The drawing under review shows one solid part. Ordinate dimensions are in mm from its lowest x, y, z. A direction names the side the tool comes from. Coordinates: 2 decimals unless noted, no trailing zeros. Order: outer loops, then holes, each group sorted by start corner. A loop starts at its lowest first (then second) coordinate and runs counter-clockwise, first axis right, second up. Notation, with made-up numbers: (-38, 25.25) -> (-15, 25.25) arc R27 ccw to (-15, 46.25) -> close; hole circle Ø1 at (-10.5, 40). An arc over 180 degrees is marked (long way). Use one line per item in the form item = value.
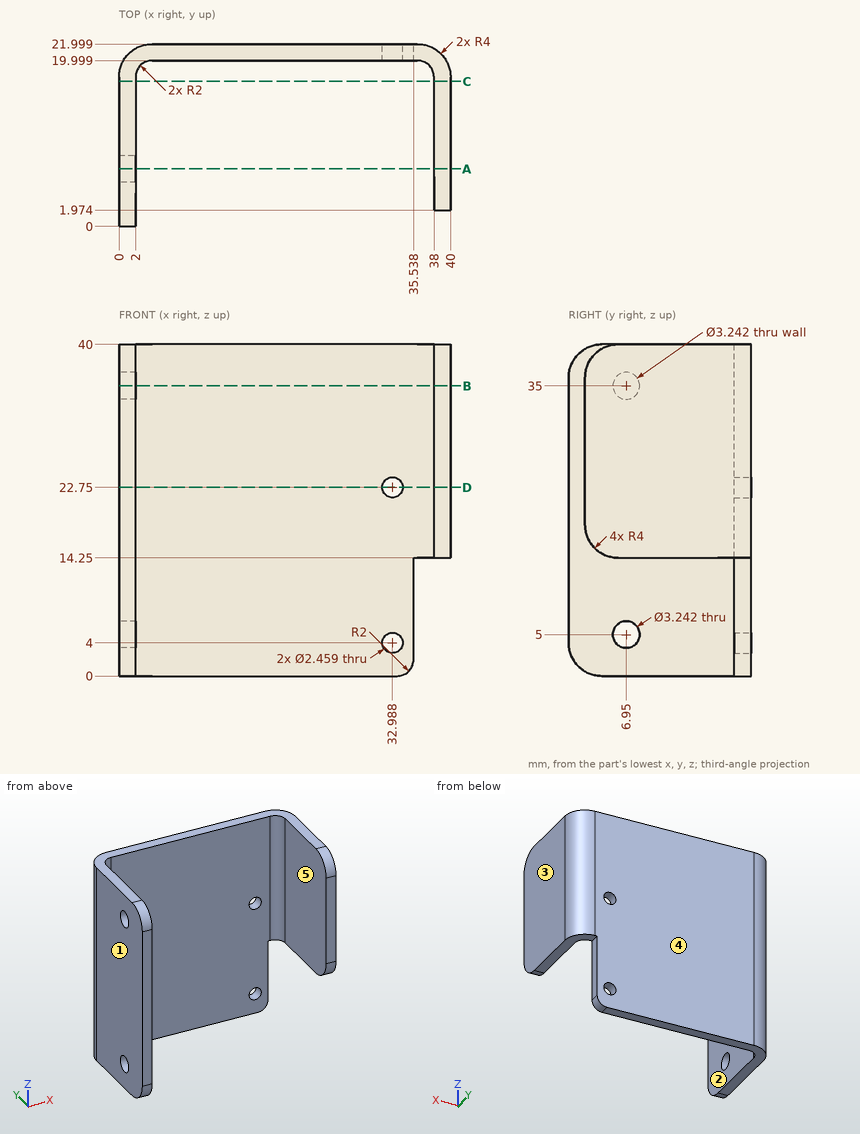
Item 1: Tool access review of the marked faces 1 and 2: name each direction out of +Z, -Z, +X, -X, +Y, -Y from which nothing blocks a thin tool from reaching the whole face with its end or side.
Results found:
face_1 = +Z, -Z, -X, +Y, -Y
face_2 = +Z, -Z, -Y
Item 2: We need section A-A (y = 6.95). Write out the cut boundary in (x, z).
Results found:
outline = (0, 0) -> (2, 0) -> (2, 3.38) -> (0, 3.38) -> close; (0, 6.62) -> (2, 6.62) -> (2, 33.38) -> (0, 33.38) -> close; (0, 36.62) -> (2, 36.62) -> (2, 40) -> (0, 40) -> close; (38, 14.25) -> (40, 14.25) -> (40, 40) -> (38, 40) -> close
Item 3: We need section C-C (y = 17.5). Write out the cut boundary in (x, z).
Results found:
outline = (0, 0) -> (2, 0) -> (2, 40) -> (0, 40) -> close; (38, 14.25) -> (40, 14.25) -> (40, 40) -> (38, 40) -> close
Item 4: We need section D-D (z = 22.75). Write out the cut boundary in (x, y).
Results found:
outline = (0, 0) -> (2, 0) -> (2, 18) arc R2 cw to (4, 20) -> (31.76, 20) -> (31.76, 22) -> (4, 22) arc R4 ccw to (0, 18) -> close; (34.22, 20) -> (36, 20) arc R2 cw to (38, 18) -> (38, 1.97) -> (40, 1.97) -> (40, 18) arc R4 ccw to (36, 22) -> (34.22, 22) -> close
Item 5: To check wall thickness, follow L1, parallel to Z at x = 1, y = 6.95; L2, parallel to X at y = 11.25, z = 15; L3, parallel to X at y = 2.25, z = 6. State the ranges of each line that lie inside material, in increasing order. Write a range as from..to.
Results found:
L1 = 0..3.38, 6.62..33.38, 36.62..40
L2 = 0..2, 38..40
L3 = 0..2
Item 6: We need section B-B (z = 35). Write out the cut boundary in (x, y).
Results found:
outline = (0, 0) -> (2, 0) -> (2, 5.33) -> (0, 5.33) -> close; (0, 8.57) -> (2, 8.57) -> (2, 18) arc R2 cw to (4, 20) -> (36, 20) arc R2 cw to (38, 18) -> (38, 1.97) -> (40, 1.97) -> (40, 18) arc R4 ccw to (36, 22) -> (4, 22) arc R4 ccw to (0, 18) -> close
Item 7: Draft analysis for pull direction X (two halves, no side actions). For the marked faces 3, 4 and 5, state which applies: released by +X, released by -X, zero draft, split by the parting line, or undercut.
Results found:
face_3 = released by +X
face_4 = zero draft
face_5 = undercut
Item 8: Clearance check with flat-ended pins moving along their axes: pin 1 (10 mm diameter, centred on x = 12, z = 17, fed in from -Y); pin 2 (3.5 mm diameter, centred on y = 6.95, z = 5, fed in from +X); pin 3 (1 mm diameter, centred on x = 38.5, z = 24, fed in from -Y). State where each tip first meets the part, or that it passes through.
Results found:
pin_1 = 20
pin_2 = 2
pin_3 = 1.97
